Part model, mm, in its own coordinate system. Face numbers are marked on the shaded views. A direction names the side the tool comes from. Give positions to 0.01 mm unless a question says otherwise; leave off trailing zeros. Loops run counter-clockwise (first coordinate to the right, second up) from the corner with the lowest first, then second, coordinate; pieces in that order, holes last. Notation, with made-up numbers: (17, 52) -> (32, 52) arc R17 cw to (32, 72) -> close; hole circle Ø2 at (-8.5, -39.5). An arc over 180 degrees is marked (long way). Write item = value, one per line.
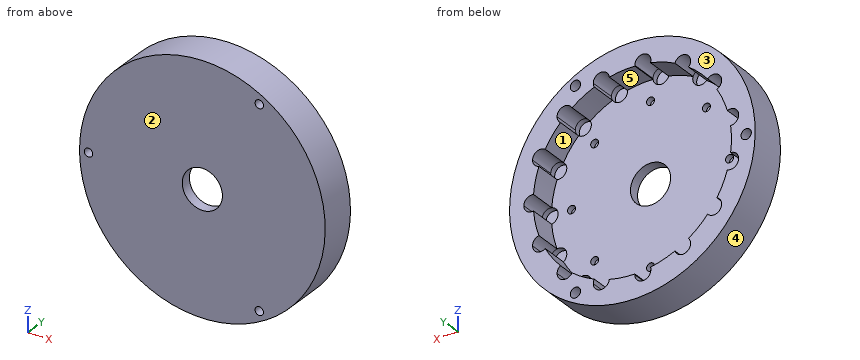
from build123d import *
from build123d.topology import SkipClean

# Parameters (mm, degrees)
SKETCH1_R           = 45.85
SKETCH1_R_2         = 7.5
SKETCH1_R_3         = 1.5635
BOSS_EXTRUDE1_DEPTH = 4
SKETCH1_6_R         = 1.48
SKETCH1_6_R_2       = 3
CUT_EXTRUDE1_DEPTH  = 2.22
BOSS_EXTRUDE2_START = 10.22
SKETCH1_7_R         = 45.85
SKETCH1_7_R_2       = 1.5635
BOSS_EXTRUDE2_DEPTH = 10.22
SKETCH2_R           = 1.925
CUT_EXTRUDE2_DEPTH  = 4


with BuildPart() as part:
    # Sketch1 → Boss-Extrude1 (new body)
    with BuildSketch(Plane(origin=(0, 0, 0), x_dir=(1, 0, 0), z_dir=(0, 1, 0))):
        with Locations(Location((0, 0, 0), (0, 0, 270))):
            Circle(SKETCH1_R)
        with Locations(Location((0, 0, 0), (0, 0, 270))):
            Circle(SKETCH1_R_2, mode=Mode.SUBTRACT)
        with Locations(Location((-42.5, 0, 0), (0, 0, 270))):
            Circle(SKETCH1_R_3, mode=Mode.SUBTRACT)
        with Locations(Location((21.25, 36.806079661, 0), (0, 0, 270))):
            Circle(SKETCH1_R_3, mode=Mode.SUBTRACT)
        with Locations(Location((21.25, -36.806079661, 0), (0, 0, 270))):
            Circle(SKETCH1_R_3, mode=Mode.SUBTRACT)
    extrude(amount=-BOSS_EXTRUDE1_DEPTH)

    # Sketch1_6 → Cut-Extrude1 (cut)
    with BuildSketch(Plane(origin=(0, 0, 0), x_dir=(1, 0, 0), z_dir=(0, 1, 0))):
        with Locations(Location((-29.5, 0, 0), (0, 0, 270))):
            Circle(SKETCH1_6_R)
        with Locations(Location((-20.859650045, 20.859650045, 0), (0, 0, 270))):
            Circle(SKETCH1_6_R)
        with Locations(Location((0, 29.5, 0), (0, 0, 270))):
            Circle(SKETCH1_6_R)
        with Locations(Location((20.859650045, 20.859650045, 0), (0, 0, 270))):
            Circle(SKETCH1_6_R)
        with Locations(Location((29.5, 0, 0), (0, 0, 270))):
            Circle(SKETCH1_6_R)
        with Locations(Location((20.859650045, -20.859650045, 0), (0, 0, 270))):
            Circle(SKETCH1_6_R)
        with Locations(Location((0, -29.5, 0), (0, 0, 270))):
            Circle(SKETCH1_6_R)
        with Locations(Location((-20.859650045, -20.859650045, 0), (0, 0, 270))):
            Circle(SKETCH1_6_R)
        with Locations(Location((-36.680535028, 7.796688406, 0), (0, 0, 270))):
            Circle(SKETCH1_6_R_2)
        with Locations(Location((-36.680535028, -7.796688406, 0), (0, 0, 270))):
            Circle(SKETCH1_6_R_2)
        with Locations(Location((-30.338137289, 22.041946961, 0), (0, 0, 270))):
            Circle(SKETCH1_6_R_2)
        with Locations(Location((-30.338137289, -22.041946961, 0), (0, 0, 270))):
            Circle(SKETCH1_6_R_2)
        with Locations(Location((-18.75, -32.475952642, 0), (0, 0, 270))):
            Circle(SKETCH1_6_R_2)
        with Locations(Location((-3.919817373, -37.294571076, 0), (0, 0, 270))):
            Circle(SKETCH1_6_R_2)
        with Locations(Location((11.588137289, -35.664619361, 0), (0, 0, 270))):
            Circle(SKETCH1_6_R_2)
        with Locations(Location((25.092397738, -27.867930955, 0), (0, 0, 270))):
            Circle(SKETCH1_6_R_2)
        with Locations(Location((34.257954662, -15.252624115, 0), (0, 0, 270))):
            Circle(SKETCH1_6_R_2)
        with Locations(Location((37.5, 0, 0), (0, 0, 270))):
            Circle(SKETCH1_6_R_2)
        with Locations(Location((34.257954662, 15.252624115, 0), (0, 0, 270))):
            Circle(SKETCH1_6_R_2)
        with Locations(Location((25.092397738, 27.867930955, 0), (0, 0, 270))):
            Circle(SKETCH1_6_R_2)
        with Locations(Location((11.588137289, 35.664619361, 0), (0, 0, 270))):
            Circle(SKETCH1_6_R_2)
        with Locations(Location((-3.919817373, 37.294571076, 0), (0, 0, 270))):
            Circle(SKETCH1_6_R_2)
        with Locations(Location((-18.75, 32.475952642, 0), (0, 0, 270))):
            Circle(SKETCH1_6_R_2)
    extrude(amount=-CUT_EXTRUDE1_DEPTH, mode=Mode.SUBTRACT)

    # Sketch1_7 → Boss-Extrude2 (add)
    with SkipClean():  # the faces are left unmerged after this step: merging them gives an invalid solid
        with BuildSketch(Plane(origin=(0, 0, 0), x_dir=(1, 0, 0), z_dir=(0, 1, 0)).offset(BOSS_EXTRUDE2_START)):
            with Locations(Location((0, 0, 0), (0, 0, 270))):
                Circle(SKETCH1_7_R)
            with Locations(Location((-42.5, 0, 0), (0, 0, 270))):
                Circle(SKETCH1_7_R_2, mode=Mode.SUBTRACT)
            with Locations(Location((21.25, -36.806079661, 0), (0, 0, 270))):
                Circle(SKETCH1_7_R_2, mode=Mode.SUBTRACT)
            with BuildLine():
                ThreePointArc((36.883333333, 2.935936345), (39.39076704, 2.32916294), (40.5, 0))
                ThreePointArc((40.5, 0), (39.39076704, -2.32916294), (36.883333333, -2.935936345))
                ThreePointArc((36.883333333, -2.935936345), (36.191461227, -7.69273256), (34.888754523, -12.319691873))
                ThreePointArc((34.888754523, -12.319691873), (36.59166411, -13.367471546), (37.257954662, -15.252624115))
                ThreePointArc((37.257954662, -15.252624115), (35.6231437, -17.924001829), (32.500448736, -17.683914497))
                ThreePointArc((32.500448736, -17.683914497), (29.933628792, -21.748054335), (26.861593101, -25.445133446))
                ThreePointArc((26.861593101, -25.445133446), (27.767055295, -26.50917897), (28.092397738, -27.867930955))
                ThreePointArc((28.092397738, -27.867930955), (25.872343464, -30.764771418), (22.497941295, -29.37418318))
                ThreePointArc((22.497941295, -29.37418318), (18.5, -32.04293994), (14.189818202, -34.170880284))
                ThreePointArc((14.189818202, -34.170880284), (14.486847583, -34.891651942), (14.588137289, -35.664619361))
                ThreePointArc((14.588137289, -35.664619361), (11.748752331, -38.660316744), (8.605335417, -35.985388734))
                ThreePointArc((8.605335417, -35.985388734), (3.867553141, -36.797310129), (-0.935505175, -36.988171489))
                ThreePointArc((-0.935505175, -36.988171489), (-0.92374189, -37.141170608), (-0.919817373, -37.294571076))
                ThreePointArc((-0.919817373, -37.294571076), (-4.385552663, -40.258199029), (-6.775211132, -36.37439366))
                ThreePointArc((-6.775211132, -36.37439366), (-11.433628792, -35.189091103), (-15.899071208, -33.409871815))
                ThreePointArc((-15.899071208, -33.409871815), (-20.25, -35.074028853), (-20.984262125, -30.47393547))
                ThreePointArc((-20.984262125, -30.47393547), (-24.757832435, -27.496358543), (-28.113543391, -24.054701786))
                ThreePointArc((-28.113543391, -24.054701786), (-32.765188272, -23.805302718), (-31.564943561, -19.304256991))
                ThreePointArc((-31.564943561, -19.304256991), (-33.801181933, -15.049255794), (-35.466928517, -10.540255288))
                ThreePointArc((-35.466928517, -10.540255288), (-39.61497783, -8.420423478), (-36.687759497, -4.796697105))
                ThreePointArc((-36.687759497, -4.796697105), (-37, 0), (-36.687759497, 4.796697105))
                ThreePointArc((-36.687759497, 4.796697105), (-39.61497783, 8.420423478), (-35.466928517, 10.540255288))
                ThreePointArc((-35.466928517, 10.540255288), (-33.801181933, 15.049255794), (-31.564943561, 19.304256991))
                ThreePointArc((-31.564943561, 19.304256991), (-32.765188272, 23.805302718), (-28.113543391, 24.054701786))
                ThreePointArc((-28.113543391, 24.054701786), (-24.757832435, 27.496358543), (-20.984262125, 30.47393547))
                ThreePointArc((-20.984262125, 30.47393547), (-20.25, 35.074028853), (-15.899071208, 33.409871815))
                ThreePointArc((-15.899071208, 33.409871815), (-11.433628792, 35.189091103), (-6.775211132, 36.37439366))
                ThreePointArc((-6.775211132, 36.37439366), (-4.385552663, 40.258199029), (-0.919817373, 37.294571076))
                ThreePointArc((-0.919817373, 37.294571076), (-0.92374189, 37.141170608), (-0.935505175, 36.988171489))
                ThreePointArc((-0.935505175, 36.988171489), (3.867553141, 36.797310129), (8.605335417, 35.985388734))
                ThreePointArc((8.605335417, 35.985388734), (11.748752331, 38.660316744), (14.588137289, 35.664619361))
                ThreePointArc((14.588137289, 35.664619361), (14.486847583, 34.891651942), (14.189818202, 34.170880284))
                ThreePointArc((14.189818202, 34.170880284), (18.5, 32.04293994), (22.497941295, 29.37418318))
                ThreePointArc((22.497941295, 29.37418318), (25.872343464, 30.764771418), (28.092397738, 27.867930955))
                ThreePointArc((28.092397738, 27.867930955), (27.767055295, 26.50917897), (26.861593101, 25.445133446))
                ThreePointArc((26.861593101, 25.445133446), (29.933628792, 21.748054335), (32.500448736, 17.683914497))
                ThreePointArc((32.500448736, 17.683914497), (35.6231437, 17.924001829), (37.257954662, 15.252624115))
                ThreePointArc((37.257954662, 15.252624115), (36.59166411, 13.367471546), (34.888754523, 12.319691873))
                ThreePointArc((34.888754523, 12.319691873), (36.191461227, 7.69273256), (36.883333333, 2.935936345))
            make_face(mode=Mode.SUBTRACT)
            with Locations(Location((21.25, 36.806079661, 0), (0, 0, 270))):
                Circle(SKETCH1_7_R_2, mode=Mode.SUBTRACT)
        extrude(amount=-BOSS_EXTRUDE2_DEPTH)

    # Sketch2 → Cut-Extrude2 (cut)
    with SkipClean():  # the faces are left unmerged after this step: merging them gives an invalid solid
        with BuildSketch(Plane(origin=(0, 10.22, 0), x_dir=(1, 0, 0), z_dir=(0, 1, 0))):
            with Locations(Location((-42.5, 0, 0), (0, 0, 270))):
                Circle(SKETCH2_R)
            with Locations(Location((21.25, 36.806079661, 0), (0, 0, 270))):
                Circle(SKETCH2_R)
            with Locations(Location((21.25, -36.806079661, 0), (0, 0, 270))):
                Circle(SKETCH2_R)
        extrude(amount=-CUT_EXTRUDE2_DEPTH, mode=Mode.SUBTRACT)


solid = part.part
1) Slice it at A-A, the plane x = -5.5. List the corners of the cut face in (y, z).
Resolved:
outline = (-4, -45.52) -> (10.22, -45.52) -> (10.22, -39.84) -> (-2.22, -39.84) -> (-2.22, -34.74) -> (0, -34.74) -> (0, -5.1) -> (-4, -5.1) -> close; (-4, 5.1) -> (0, 5.1) -> (0, 34.74) -> (-2.22, 34.74) -> (-2.22, 39.84) -> (10.22, 39.84) -> (10.22, 45.52) -> (-4, 45.52) -> close
2) Pull direction X, two halves, no side cores. Call the marked faces 3, 4 and 5: pulls with the +X half, pulls with the -X half, needs draft (parallel to the pull), parting line crosses it, or undercut.
Resolved:
face_3 = needs draft
face_4 = parting line crosses it
face_5 = undercut
3) Which spindle directions (+Z, -Z, +X, -X, +Y, -Y) get a long thin tool onto all of the face, cutting with end or side? Do the marked faces 1 and 2. Say none if no direction does.
Resolved:
face_1 = +Y
face_2 = +Z, -Z, +X, -X, -Y
4) Drill centre lines: line 1 along X through (y, z) = (8, 24.5); line 2 along X through (y, z) = (8.25, -33.5); line 3 along Y through (x, z) = (-4.5, 16). Where is each one in solid material? Low to high. Write a range as [from, to].
Resolved:
line_1 = [-38.76, -32.06], [-28.62, -27.73], [27.73, 38.76]
line_2 = [-31.3, -21.57], [-15.93, -15.71], [15.71, 31.3]
line_3 = [-4, 0]
5) Drop flat-ended pins along their axis: P1, Ø3.5, axis at x = 0, z = -29.5, coming from the +Y side; P2, Ø6.5, axis at x = 34.5, z = -14, coming from the +Y side; P3, Ø5, axis at x = -35.5, y = 8.5, coming from the +Z side; P4, Ø0.9, axis at x = 21, z = 20.5, coming from the +Y side. Give the stop position or say it passes through.
Resolved:
P1 = 0
P2 = 10.22
P3 = 31.83
P4 = -2.22
6) Slice it at C-C, the plane x = 18. List the corners of the cut face in (y, z).
Resolved:
outline = (-4, -42.17) -> (10.22, -42.17) -> (10.22, -32.33) -> (0, -32.33) -> (0, 32.33) -> (10.22, 32.33) -> (10.22, 42.17) -> (-4, 42.17) -> close
7) Slice it at B-B, the plane y = 8. Count the separate pieces of the cut face and the enclosed holes in it, and give its area (3 significant figures).
Resolved:
separate_pieces = 1
enclosed_holes = 4
area = 2,010 mm²
